from build123d import *

# Parameters (mm, degrees)
SKETCH1_R           = 51
BOSS_EXTRUDE1_DEPTH = 13.5
SHELL1_T            = -7
SKETCH2_R           = 18.5
CUT_EXTRUDE1_DEPTH  = 7
SKETCH3_R           = 23.6
CUT_EXTRUDE2_DEPTH  = 3
SKETCH5_R           = 1.6
CUT_EXTRUDE3_DEPTH  = 13.5
SKETCH6_R           = 2.25
CUT_EXTRUDE4_DEPTH  = 6


with BuildPart() as part:
    # Sketch1 → Boss-Extrude1 (new body)
    with BuildSketch(Plane.XY):
        Circle(SKETCH1_R)
    extrude(amount=BOSS_EXTRUDE1_DEPTH)

    # Shell1
    shell1_openings = [part.faces().sort_by_distance(p)[0] for p in [
        (0, 0, 13.5),
    ]]
    offset(amount=SHELL1_T, openings=shell1_openings, kind=Kind.INTERSECTION)

    # Sketch2 → Cut-Extrude1 (cut)
    with BuildSketch(Plane(origin=(0, 0, 0), x_dir=(-1, 0, 0), z_dir=(0, 0, -1))):
        Circle(SKETCH2_R)
    extrude(amount=-CUT_EXTRUDE1_DEPTH, mode=Mode.SUBTRACT)

    # Sketch3 → Cut-Extrude2 (cut)
    with BuildSketch(Plane.XY.offset(7)):
        Circle(SKETCH3_R)
    extrude(amount=-CUT_EXTRUDE2_DEPTH, mode=Mode.SUBTRACT)

    # Sketch5 → Cut-Extrude3 (cut)
    with BuildSketch(Plane.XY.offset(13.5)):
        with Locations((0, 47.5)):
            Circle(SKETCH5_R)
        with Locations((47.5, 0)):
            Circle(SKETCH5_R)
        with Locations((0, -47.5)):
            Circle(SKETCH5_R)
        with Locations((-47.5, 0)):
            Circle(SKETCH5_R)
    extrude(amount=-CUT_EXTRUDE3_DEPTH, mode=Mode.SUBTRACT)

    # Sketch6 → Cut-Extrude4 (cut)
    with BuildSketch(Plane(origin=(0, 0, 0), x_dir=(-1, 0, 0), z_dir=(0, 0, -1))):
        with Locations((-33.587572106, 33.587572106)):
            Circle(SKETCH6_R)
        with Locations((33.587572106, 33.587572106)):
            Circle(SKETCH6_R)
        with Locations((33.587572106, -33.587572106)):
            Circle(SKETCH6_R)
        with Locations((-33.587572106, -33.587572106)):
            Circle(SKETCH6_R)
    extrude(amount=-CUT_EXTRUDE4_DEPTH, mode=Mode.SUBTRACT)


solid = part.part
Could you check a few things on this model? Use its own coordinates, in mm. A direction names the side the tool comes from. Coordinates: 2 decimals unless noted, no trailing zeros. Order: outer loops, then holes, each group sorted by start corner. A loop starts at its lowest first (then second) coordinate and runs counter-clockwise, first axis right, second up.
Q1. Please list where these lines run through material, in increasing order: L1, parallel to Y at x = 0, z = 6.05; L2, parallel to Y at x = 35, z = 8.5; L3, parallel to X at y = -19.5, z = 12.
Q2. Will these pins go through, and if not, where does the flat tip stop? pin 1 (4 mm diameter, centred on x = -21, z = 2.5, fed in from +Y); pin 2 (2.5 mm diameter, centred on x = -47.5, y = 0, fed in from +Z); pin 3 (1.3 mm diameter, centred on x = 33.5, y = -34.5, fed in from -Z); pin 4 (1 mm diameter, centred on x = -24.5, z = 7, fed in from +Y).
Q3. Suppose I cut it at D-D on y = -11.5. Please give me the cut outline in (x, z), and give its area (3 significant figures).
Q4. Thinking about a two-plate mould opening in Y: for faces 1 (the flat face through (-23, 38, 13.5)), 2 (the cylindrical face through (35.37, -34.96, 2.96)), 3 (the cylindrical face through (-9.538, -42.954, 10.204)), which applies, released by +Y, released by -Y, zero draft, split by the parting line, or undercut?
Q5. Which directions (+Z, -Z, +X, -X, +Y, -Y) give clear straight access to the entire face, cutting with the end or side of a thin tool? Please do faces 4 (the flat face through (10, -16, 4)), 5 (the cylindrical face through (0.74, -48.92, 6.84)), 6 (the flat face through (-34, -34, 6)).
Q6. Suppose I cut it at A-A on x = 0. Please give me the cut outline in (y, z), and give its area (3 significant figures).
Q7. Suppose I cut it at C-C on z = 12. Please give me the cut outline in (x, y).
Answer:
1. L1: y = -51 to -49.1, -45.9 to -23.6, 23.6 to 45.9, 49.1 to 51
1. L2: y = -37.09 to -26.66, 26.66 to 37.09
1. L3: x = -47.12 to -39.44, 39.44 to 47.12
2. pin 1: stops at y = 47.33
2. pin 2: passes through
2. pin 3: stops at z = 6
2. pin 4: stops at y = 45
3. outline: (-49.69, 0) - (-14.49, 0) - (-14.49, 4) - (-20.61, 4) - (-20.61, 7) - (-42.47, 7) - (-42.47, 13.5) - (-49.69, 13.5) - close; (14.49, 0) - (49.69, 0) - (49.69, 13.5) - (42.47, 13.5) - (42.47, 7) - (20.61, 7) - (20.61, 4) - (14.49, 4) - close
3. area: 550 mm2
4. face 1: zero draft
4. face 2: undercut
4. face 3: undercut
5. face 4: +Z
5. face 5: +Z, -Z
5. face 6: -Z
6. outline: (-51, 0) - (-49.1, 0) - (-49.1, 13.5) - (-51, 13.5) - close; (-45.9, 0) - (-18.5, 0) - (-18.5, 4) - (-23.6, 4) - (-23.6, 7) - (-44, 7) - (-44, 13.5) - (-45.9, 13.5) - close; (18.5, 0) - (45.9, 0) - (45.9, 13.5) - (44, 13.5) - (44, 7) - (23.6, 7) - (23.6, 4) - (18.5, 4) - close; (49.1, 0) - (51, 0) - (51, 13.5) - (49.1, 13.5) - close
6. area: 429 mm2
7. outline: circle Ø102 at (0, 0); hole circle Ø3.2 at (-47.5, 0); hole circle Ø88 at (0, 0); hole circle Ø3.2 at (0, -47.5); hole circle Ø3.2 at (0, 47.5); hole circle Ø3.2 at (47.5, 0)
